Part model, mm, in its own coordinate system. Face numbers are marked on the shaded views. A direction names the side the tool comes from. Coordinates: 2 decimals unless noted, no trailing zeros. Loops run counter-clockwise (first coordinate to the right, second up) from the corner with the lowest first, then second, coordinate; pieces in that order, holes last. Notation, with made-up numbers: (48.5, -18.5) - (56.5, -18.5) arc R36 ccw to (56.5, 18.5) - close; hole circle Ø5 at (22.25, -25). An arc over 180 degrees is marked (long way). Use a Markdown table: item, result. Add a question column.
1) Drop flat-ended pins along their axis: P1, Ø3, axis at x = 1, z = 1.5, coming from the +Y side; P2, Ø1.9, axis at y = 3.5, z = 6, coming from the +X side (3 decimals); P3, Ø8, axis at x = 44.5, y = 8, coming from the -Z side. Give the stop position or say it passes through.
2) Band-saw the part on D-D (x = 30). Give the cut face in (y, z).
3) Probe probe 1 along X at (y, z) = (1.35, 0) (3 decimals); probe 2 along Z at (x, y) = (0, 0.7) (3 decimals); probe 3 along X at (y, z) = (9, 8.25). List the from-to ranges inside material, lowest first. Write a range as [from, to].
4) Pull direction X, two halves, no side cores. Call the marked faces 1 and 2: +X half, -X half, draft (parallel to the pull), parting line (faces both ways), or undercut.
5) Band-saw the part on C-C (z = -0.75). Give the cut face in (x, y).
6) Band-saw the part on B-B (z = 5.5). Give the cut face in (x, y) (3 decimals).
7) Band-saw the part on A-A (y = 7.5). Give the cut face in (x, z).
8) Tool access for the marked faces 3 and 4: list every direction of +Z, -Z, +X, -X, +Y, -Y with a clear straight run to the whole face (end or side of a thin tool).
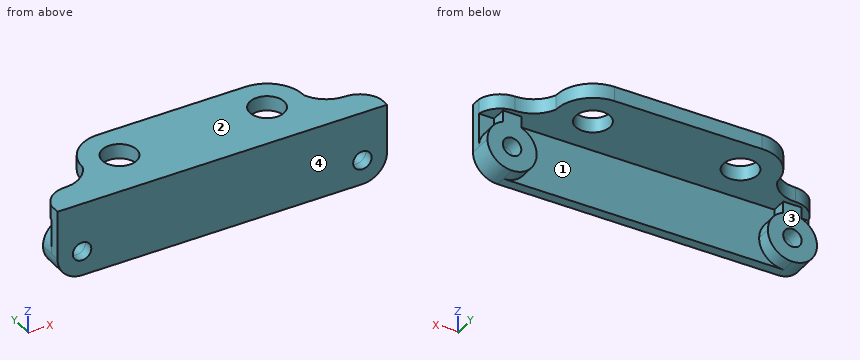
from build123d import *

# Parameters (mm, degrees)
SKETCH1_R           = 1.875
BOSS_EXTRUDE1_DEPTH = 2
SKETCH2_W           = 3.125
SKETCH2_H           = 3
SKETCH2_W_2         = 3.75
SKETCH2_W_3         = 26.625
BOSS_EXTRUDE2_DEPTH = 3
SKETCH3_W           = 67
SKETCH3_H           = 3
BOSS_EXTRUDE3_DEPTH = 20
CUT_EXTRUDE1_REACH  = 70.513
SKETCH4_R           = 3.5


with BuildPart() as part:
    # Sketch1 → Boss-Extrude1 (new body)
    with BuildSketch(Plane(origin=(0, 0, 0), x_dir=(1, 0, 0), z_dir=(0, 1, 0))):
        with BuildLine():
            Line((0, 5), (57, 5))
            ThreePointArc((57, 5), (60.535533906, 3.535533906), (62, 0))
            Line((62, 0), (62, -10))
            Line((62, -10), (-5, -10))
            Line((-5, -10), (-5, 0))
            ThreePointArc((-5, 0), (-3.535533906, 3.535533906), (0, 5))
        make_face()
        with Locations(Location((0, 0, 0), (0, 0, 270))):
            Circle(SKETCH1_R, mode=Mode.SUBTRACT)
        with Locations(Location((57, 0, 0), (0, 0, 270))):
            Circle(SKETCH1_R, mode=Mode.SUBTRACT)
    extrude(amount=BOSS_EXTRUDE1_DEPTH)

    # Sketch2 → Boss-Extrude2 (add)
    with BuildSketch(Plane(origin=(0, 2, 0), x_dir=(1, 0, 0), z_dir=(0, 1, 0))):
        with BuildLine():
            ThreePointArc((0, 5), (-3.535533906, 3.535533906), (-5, 0))
            ThreePointArc((-5, 0), (-4.145780988, -2.795084972), (-1.875, -4.635124054))
            Line((-1.875, -4.635124054), (-1.875, 0))
            ThreePointArc((-1.875, 0), (0, 1.875), (1.875, 0))
            Line((1.875, 0), (1.875, -4.635124054))
            ThreePointArc((1.875, -4.635124054), (4.145780988, -2.795084972), (5, 0))
            ThreePointArc((5, 0), (3.535533906, 3.535533906), (0, 5))
        make_face()
        with BuildLine():
            Line((-1.875, 0), (-1.875, -4.635124054))
            ThreePointArc((-1.875, -4.635124054), (0, -5), (1.875, -4.635124054))
            Line((1.875, -4.635124054), (1.875, 0))
            ThreePointArc((1.875, 0), (0, -1.875), (-1.875, 0))
        make_face()
        with BuildLine():
            Line((-1.875, -4.635124054), (-1.875, -7))
            Line((-1.875, -7), (1.875, -7))
            Line((1.875, -7), (1.875, -4.635124054))
            ThreePointArc((1.875, -4.635124054), (0, -5), (-1.875, -4.635124054))
        make_face()
        with Locations((-3.4375, -8.5)):
            Rectangle(SKETCH2_W, SKETCH2_H)
        with Locations((0, -8.5)):
            Rectangle(SKETCH2_W_2, SKETCH2_H)
        with Locations((15.1875, -8.5)):
            Rectangle(SKETCH2_W_3, SKETCH2_H)
        with BuildLine():
            ThreePointArc((57, 5), (52.092066613, 0.955086312), (55.125, -4.635124054))
            Line((55.125, -4.635124054), (55.125, 0))
            ThreePointArc((55.125, 0), (57, 1.875), (58.875, 0))
            Line((58.875, 0), (58.875, -4.635124054))
            ThreePointArc((58.875, -4.635124054), (61.145780988, -2.795084972), (62, 0))
            ThreePointArc((62, 0), (60.535533906, 3.535533906), (57, 5))
        make_face()
        with BuildLine():
            Line((55.125, 0), (55.125, -4.635124054))
            ThreePointArc((55.125, -4.635124054), (57, -5), (58.875, -4.635124054))
            Line((58.875, -4.635124054), (58.875, 0))
            ThreePointArc((58.875, 0), (57, -1.875), (55.125, 0))
        make_face()
        with BuildLine():
            Line((55.125, -4.635124054), (55.125, -7))
            Line((55.125, -7), (58.875, -7))
            Line((58.875, -7), (58.875, -4.635124054))
            ThreePointArc((58.875, -4.635124054), (57, -5), (55.125, -4.635124054))
        make_face()
        with Locations((60.4375, -8.5)):
            Rectangle(SKETCH2_W, SKETCH2_H)
        with Locations((57, -8.5)):
            Rectangle(SKETCH2_W_2, SKETCH2_H)
        with Locations((41.8125, -8.5)):
            Rectangle(SKETCH2_W_3, SKETCH2_H)
    extrude(amount=BOSS_EXTRUDE2_DEPTH)

    # Sketch3 → Boss-Extrude3 (add)
    with BuildSketch(Plane(origin=(0, 5, 0), x_dir=(1, 0, 0), z_dir=(0, 1, 0))):
        with Locations((28.5, -8.5)):
            Rectangle(SKETCH3_W, SKETCH3_H)
    extrude(amount=BOSS_EXTRUDE3_DEPTH)

    # Sketch4 → Cut-Extrude1 (cut, up to next)
    with BuildSketch(Plane.XY.offset(10), mode=Mode.PRIVATE) as cut_extrude1_sk1:
        with BuildLine():
            ThreePointArc((-5, 2), (-3.201562119, 4.876952648), (0, 6))
            ThreePointArc((0, 6), (3.605551275, 7.091673087), (6, 10))
            ThreePointArc((6, 10), (8.196699141, 15.303300859), (13.5, 17.5))
            Line((13.5, 17.5), (43.5, 17.5))
            ThreePointArc((43.5, 17.5), (48.803300859, 15.303300859), (51, 10))
            ThreePointArc((51, 10), (53.394448725, 7.091673087), (57, 6))
            ThreePointArc((57, 6), (60.201562119, 4.876952648), (62, 2))
            Line((62, 2), (62, 25))
            Line((62, 25), (-5, 25))
            Line((-5, 25), (-5, 2))
        make_face()
    cut_extrude1_tool1 = extrude(cut_extrude1_sk1.sketch, amount=-CUT_EXTRUDE1_REACH, mode=Mode.PRIVATE) & part.part
    # Sketch4 → Cut-Extrude1 (cut, up to next)
    with BuildSketch(Plane.XY.offset(10), mode=Mode.PRIVATE) as cut_extrude1_sk2:
        with Locations((13.5, 10)):
            Circle(SKETCH4_R)
    cut_extrude1_tool2 = extrude(cut_extrude1_sk2.sketch, amount=-CUT_EXTRUDE1_REACH, mode=Mode.PRIVATE) & part.part
    # Sketch4 → Cut-Extrude1 (cut, up to next)
    with BuildSketch(Plane.XY.offset(10), mode=Mode.PRIVATE) as cut_extrude1_sk3:
        with Locations((43.5, 10)):
            Circle(SKETCH4_R)
    cut_extrude1_tool3 = extrude(cut_extrude1_sk3.sketch, amount=-CUT_EXTRUDE1_REACH, mode=Mode.PRIVATE) & part.part
    add(cut_extrude1_tool1.solids().sort_by_distance((28.5, 18.015348, 10))[0], mode=Mode.SUBTRACT)
    add(cut_extrude1_tool2.solids().sort_by_distance((13.5, 10, 10))[0], mode=Mode.SUBTRACT)
    add(cut_extrude1_tool3.solids().sort_by_distance((43.5, 10, 10))[0], mode=Mode.SUBTRACT)


solid = part.part
Answer block:
| question | item | result |
|---|---|---|
| 1 | P1 | y = 5 |
| 1 | P2 | x = 58.875 |
| 1 | P3 | z = 7 |
| 2 | outline | (0, -5) - (2, -5) - (2, 7) - (17.5, 7) - (17.5, 10) - (0, 10) - close |
| 3 | probe 1 | [-5, -1.875], [1.875, 55.125], [58.875, 62] |
| 3 | probe 2 | [-5, -1.875], [1.875, 10] |
| 3 | probe 3 | [5.48, 10.15], [16.85, 40.15], [46.85, 51.52] |
| 4 | face 1 | undercut |
| 4 | face 2 | draft |
| 5 | outline | (-4.94, 0) - (-1.72, 0) - (-1.72, 5) - (-4.94, 5) - close; (1.72, 0) - (55.28, 0) - (55.28, 5) - (52.06, 5) - (52.06, 2) - (4.94, 2) - (4.94, 5) - (1.72, 5) - close; (58.72, 0) - (61.94, 0) - (61.94, 5) - (58.72, 5) - close |
| 6 | outline | (-5, 0) - (62, 0) - (62, 2) - (58.875, 2) - (58.875, 5) - (55.125, 5) - (55.125, 2) - (1.875, 2) - (1.875, 5) - (-1.875, 5) - (-1.875, 2) - (-5, 2) - close |
| 7 | outline | (4.15, 7) - (11.05, 7) - (11.05, 10) - (4.15, 10) - close; (15.95, 7) - (41.05, 7) - (41.05, 10) - (15.95, 10) - close; (45.95, 7) - (52.85, 7) - (52.85, 10) - (45.95, 10) - close |
| 8 | face 3 | -Z, +X, -X, +Y |
| 8 | face 4 | +Z, -Z, +X, -X, -Y |
